The listing builds one solid part. Answer for the finished solid, in the listing's coordinates (mm). A direction names the side the tool comes from. Give positions to 0.01 mm unless a question says otherwise; leave off trailing zeros. Order: outer loops, then holes, each group sorted by start corner. A loop starts at its lowest first (then second) coordinate and runs counter-clockwise, first axis right, second up. Notation, with made-up numbers: (60.5, 50) - (86.5, 50) arc R29 cw to (86.5, 79) - close; hole circle Ø5 at (-20.5, 64.5). An arc over 180 degrees is marked (long way). Use a Markdown table: item, result. Add a question column.
1) Straight lines are drawn through the part: line 1 (Z direction, x = 6, y = 10); line 2 (Z direction, x = -58.5, y = 4); line 3 (X direction, y = 72, z = 32.5). For each, find the intervals that lie inside material, in ascending order.
2) Find section A-A, the plane y = 68. Determine the outline of the cut face in (x, z), plus the area to 3 significant figures.
3) The mould has two halves that part along X. Classify faces 4 (the face through (-11.536, 74.66, 51.948)), 5 (the face through (-17, 55.118, -33)), 6 (the face through (-55.118, -17, 33)): released by +X, released by -X, zero draft, split by the parting line, or undercut.
4) Flat-ended cylindrical pins translate along their axes: pin 1 (6 mm diameter, centred on x = -23.5, y = -27, fed in from -Z); pin 2 (2 mm diameter, centred on x = 13.5, z = -34.5, fed in from +Y); pin 3 (2 mm diameter, centred on x = -49, y = 32.5, fed in from +Z). Find the tip coordinate at first contact, or state that the pin passes through.
5) For faces 1 (the face through (-12, 93.662, -44)), 2 (the face through (-74.7, 35.3, 27.1)), 3 (the face through (-35.31, 74.12, 27.08)), determine the directions among +Z, -Z, +X, -X, +Y, -Y from which every point of the face is accessible in a straight line to the end or side of a thin tool.
from build123d import *

# Parameters (mm, degrees)
SKETCH3_R   = 53.213
SKETCH3_R_2 = 36.83


with BuildPart() as part:
    # Sketch1 → Revolve1 (revolve)
    with BuildSketch(Plane.XY):
        Polygon((-93.6625, -53.213), (-55.118, -53.213), (-55.118, -44.3484), (-93.6625, -44.6532), align=None)
    revolve(axis=Axis((-93.6625, 0, 0), (1, 0, 0)))



with BuildPart() as body_2:
    # Sketch2 → Revolve2 (revolve)
    with BuildSketch(Plane.XY):
        Polygon((44.6532, 93.6625), (44.3484, 55.118), (53.213, 55.118), (53.213, 93.6625), align=None)
    revolve(axis=Axis((0, 0, 0), (0, 1, 0)))


with BuildPart() as part_1:
    add(part.part)

    add(body_2.part)  # Sweep1 merges body 2
    # Sweep1: sweep along a path in Sketch4
    with BuildLine(Plane.XY) as sweep1_path:
        ThreePointArc((-55.118, 0), (-16.143688435, 16.143688435), (0, 55.118))
    # Sketch3 → Sweep1 (sweep)
    with BuildSketch(Plane(origin=(-55.118, 0, 0), x_dir=(0, 0, -1), z_dir=(1, 0, 0))):
        Circle(SKETCH3_R)
        Circle(SKETCH3_R_2, mode=Mode.SUBTRACT)
    sweep(path=sweep1_path.line)


solid = part_1.part
The answers:
| question | item | result |
|---|---|---|
| 1 | line 1 | -48.96 to -30.36, 30.36 to 48.96 |
| 1 | line 2 | -53.06 to -44.19, 44.19 to 53.06 |
| 1 | line 3 | -42.14 to -30.37, 30.37 to 42.14 |
| 2 | outline | circle Ø106.43 at (0, 0); hole circle Ø88.9 at (0, 0) |
| 2 | area | 2,690 mm2 |
| 3 | face 4 | split by the parting line |
| 3 | face 5 | undercut |
| 3 | face 6 | released by -X |
| 4 | pin 1 | z = -44.03 |
| 4 | pin 2 | y = 55.12 |
| 4 | pin 3 | z = 43.47 |
| 5 | face 1 | +Z, -Z, +X, -X, +Y |
| 5 | face 2 | -X |
| 5 | face 3 | +Y |
